Source: three-view drawing plus pictorial views. Frame: mm from the lowest corner of the part. A direction names the side the tool comes from. Coordinates: 2 decimals unless noted, no trailing zeros. Order: outer loops, then holes, each group sorted by start corner. A loop starts at its lowest first (then second) coordinate and runs counter-clockwise, first axis right, second up. Notation, with made-up numbers: (-23, 24) -> (9, 24) arc R12 cw to (9, 30) -> close; hole circle Ø9 at (73.5, 54). An arc over 180 degrees is marked (long way). Use one line per item in the form item = value. Start each with the question number.
1) Pin query (flat end, axial travel): pin 1 (2.5 mm diameter, centred on x = 40.26, y = 28.175, fed in from +Z); pin 2 (6.5 mm diameter, centred on y = 37.5, z = 18.5, fed in from +X) (3 decimals); pin 3 (5 mm diameter, centred on x = 17.01, y = 41.6, fed in from +Z); pin 4 (4.5 mm diameter, centred on x = 57.26, z = 30.5, fed in from +Y) (1 decimal). Return the tip coordinate at first contact, or that it passes through.
2) Ray query, line 1 along Y through (x, z) = (17, 16) (1 decimal); line 2 along Z through (x, y) = (7.5, 25); line 3 along Y through (x, z) = (30, 25) (1 decimal). Return the intervals inside material, ascending.
3) Section query A-A on z = 30.5. Output: boundary loops of the cut face in (x, y) (1 decimal).
4) Section query B-B on x = 57.26. Count the separate pieces of the cut face and the enclosed holes in it, then the cut area to 3 significant figures.
5) Draft query along Y for the marked faces 4, 5 and 6. Return one class per face: pulls with the +Y half, pulls with the -Y half, needs draft (parallel to the pull), parting line crosses it, or undercut.
6) Access query for the marked faces 1, 2 and 3. Directions: +Z, -Z, +X, -X, +Y, -Y. A direction counts if a zero-diameter tool reaches every point of the face in a straight line with its end or side. Return the directions, or none.
7) Section query D-D on z = 16. Output: boundary loops of the cut face in (x, y) (1 decimal).
8) Section query C-C on x = 24.76. Output: boundary loops of the cut face in (y, z) (1 decimal).
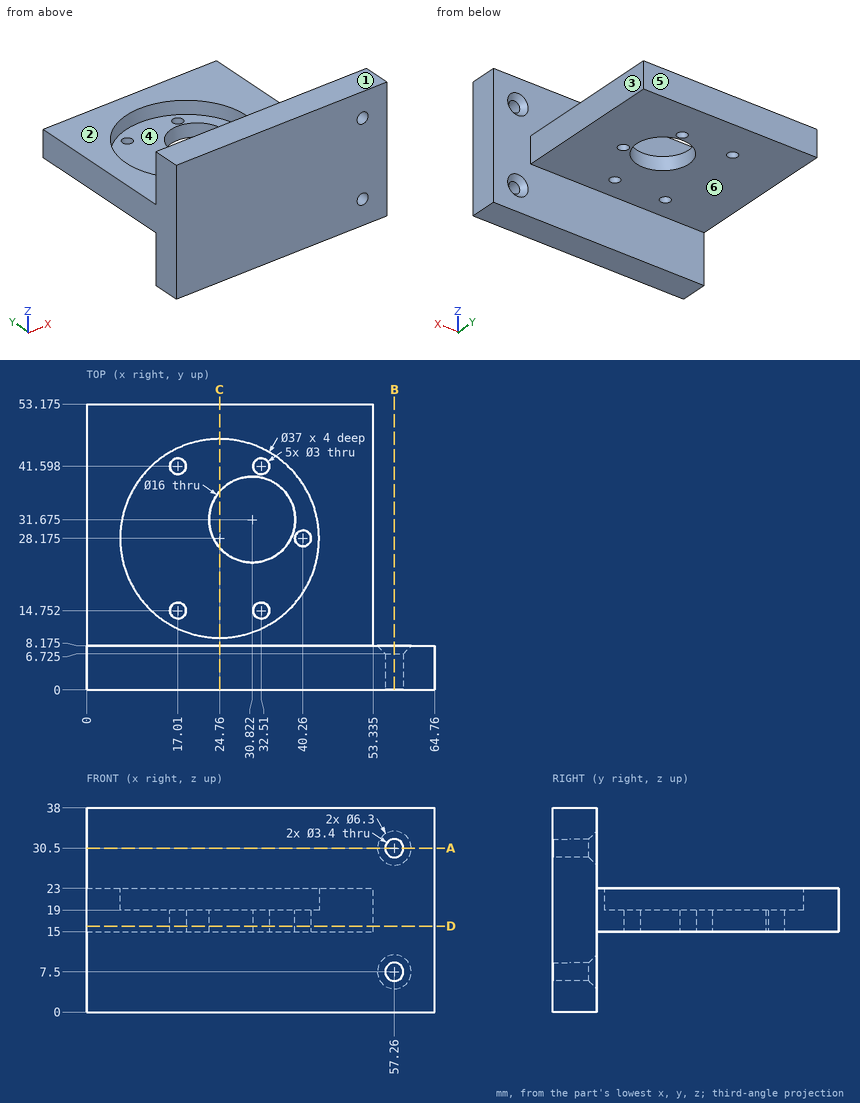
Answers below:
q1.pin_1 = through
q1.pin_2 = 53.335
q1.pin_3 = 19
q1.pin_4 = 7.3
q2.line_1 = 0 to 13.3, 16.3 to 40.1, 43.1 to 53.2
q2.line_2 = 15 to 19
q2.line_3 = 0 to 8.2
q3.outline = (0, 0) -> (55.6, 0) -> (55.6, 6.7) -> (54.1, 8.2) -> (0, 8.2) -> close; (59, 0) -> (64.8, 0) -> (64.8, 8.2) -> (60.4, 8.2) -> (59, 6.7) -> close
q4.separate_pieces = 3
q4.enclosed_holes = 0
q4.area = 251 mm^2
q5.face_4 = undercut
q5.face_5 = pulls with the +Y half
q5.face_6 = needs draft
q6.face_1 = +Z, +X, -X, +Y, -Y
q6.face_2 = +Z, +X, -X, +Y
q6.face_3 = +Z, -Z, +X, +Y
q7.outline = (0, 0) -> (64.8, 0) -> (64.8, 8.2) -> (53.3, 8.2) -> (53.3, 53.2) -> (0, 53.2) -> close; hole circle Ø3 at (17, 14.8); hole circle Ø3 at (17, 41.6); hole circle Ø16 at (30.8, 31.7); hole circle Ø3 at (32.5, 14.8); hole circle Ø3 at (32.5, 41.6); hole circle Ø3 at (40.3, 28.2)
q8.outline = (0, 0) -> (8.2, 0) -> (8.2, 15) -> (26.5, 15) -> (26.5, 19) -> (9.7, 19) -> (9.7, 23) -> (8.2, 23) -> (8.2, 38) -> (0, 38) -> close; (36.9, 15) -> (53.2, 15) -> (53.2, 23) -> (46.7, 23) -> (46.7, 19) -> (36.9, 19) -> close
